from build123d import *

# Parameters (mm, degrees)
F0_W     = 40.64
F0_H     = 40.64
F1_DEPTH = 68.58
F2_W     = 25.4
F2_H     = 40.64
F3_DEPTH = 17.78
F4_W     = 25.4
F4_H     = 17.78
F5_DEPTH = 25.4


with BuildPart() as f1:
    # F0 (on Right) → F1 (new body)
    with BuildSketch(Plane.YZ):
        with Locations((-38.1975453347, 20.5620517739)):
            Rectangle(F0_W, F0_H)
    extrude(amount=-F1_DEPTH)

    # F2 (on face) → F3 (join)
    with BuildSketch(Plane.XZ.offset(58.5175453347)):
        with Locations((-30.48, 20.5620517739)):
            Rectangle(F2_W, F2_H)
    extrude(amount=F3_DEPTH)

    # F4 (on face) → F5 (join)
    with BuildSketch(Plane(origin=(0, 0, 0.2420517739), x_dir=(1, 0, 0), z_dir=(0, 0, -1))):
        with Locations((-30.48, 67.4075453347)):
            Rectangle(F4_W, F4_H)
    extrude(amount=F5_DEPTH)


solid = f1.part
The listing builds one solid part. Answer for the finished solid, in the listing's coordinates (mm). A direction names the side the tool comes from. Give positions to 0.01 mm unless a question says otherwise; leave off trailing zeros. Loops run counter-clockwise (first coordinate to the right, second up) from the corner with the lowest first, then second, coordinate; pieces in that order, holes last. Notation, with made-up numbers: (89, 64) - (139, 64) arc R15 cw to (139, 69) - close; hole circle Ø11 at (83, 70.5). An arc over 180 degrees is marked (long way). Answer as a JSON object with one key per item and string values.
1. A cutting plane is placed at B-B (y = -53). Write down the section's boundary in (x, z).
Determined:
{"outline": "(-68.58, 0.24) - (0, 0.24) - (0, 40.88) - (-68.58, 40.88) - close"}
2. Flat-ended cylindrical pins translate along their axes: pin 1 Ø14 at (x, z) = (-7, 24.5) entering from -Y; pin 2 Ø1.5 at (y, z) = (-61.5, 9) entering from +X; pin 3 Ø20.5 at (x, y) = (-30, -34.5) entering from -Z. Find the tip coordinate at first contact, or state that the pin passes through.
Determined:
{"pin 1": "y = -58.52", "pin 2": "x = -17.78", "pin 3": "z = 0.24"}
3. A cutting plane is placed at D-D (z = -14.5). Write down the section's boundary in (x, y), then the cut area to 3 significant figures.
Determined:
{"outline": "(-43.18, -76.3) - (-17.78, -76.3) - (-17.78, -58.52) - (-43.18, -58.52) - close", "area": "452 mm²"}
4. A cutting plane is placed at A-A (z = 8). Write down the section's boundary in (x, y).
Determined:
{"outline": "(-68.58, -58.52) - (-43.18, -58.52) - (-43.18, -76.3) - (-17.78, -76.3) - (-17.78, -58.52) - (0, -58.52) - (0, -17.88) - (-68.58, -17.88) - close"}
5. A cutting plane is placed at C-C (x = -19.5). Write down the section's boundary in (y, z), then the cut area to 3 significant figures.
Determined:
{"outline": "(-76.3, -25.16) - (-58.52, -25.16) - (-58.52, 0.24) - (-17.88, 0.24) - (-17.88, 40.88) - (-76.3, 40.88) - close", "area": "2,830 mm²"}
6. For faces 1 (the flat face through (-34, -38, 0.242)), 2 (the flat face through (-56, -58.518, 20)), 3 (the flat face through (-31, -76.298, 8)), 4 (the flat face through (-34, -17.878, 20)), 5 (the flat face through (-17.78, -67, 8)), determine the directions among +Z, -Z, +X, -X, +Y, -Y from which every point of the face is accessible in a straight line to the end or side of a thin tool.
Determined:
{"face 1": "-Z, +X, -X, +Y", "face 2": "+Z, -Z, -X, -Y", "face 3": "+Z, -Z, +X, -X, -Y", "face 4": "+Z, -Z, +X, -X, +Y", "face 5": "+Z, -Z, +X, -Y"}
7. Find the intervals of material crossed by L1, parallel to Z at x = -46, y = -30.5; L2, parallel to Y at x = -13.5, z = 9; L3, parallel to X at y = -64, z = -2.5, in increasing order. Write a range as [from, to].
Determined:
{"L1": "[0.24, 40.88]", "L2": "[-58.52, -17.88]", "L3": "[-43.18, -17.78]"}
